Build history of the part. All positions in model axes, mm. Face numbers are marked on the shaded views. A direction names the side the tool comes from. Round coordinates to 2 decimals unless told otherwise and drop trailing zeros. Write each loop counter-clockwise with the first axis right and the second up, starting at its lowest first coordinate (ties: lowest second). Pieces come first, ordered by that corner, then holes. Notation, with made-up numbers: (40, -31) -> (99, -31) arc R30 cw to (99, -2) -> close; hole circle Ø5 at (21, -9.5). An arc over 180 degrees is marked (long way). Answer as CSV lines item,"result".
from build123d import *

# Parameters (mm, degrees)
BOSS_EXTRU_1_DEPTH = 10
ESQUISSE3_R        = 4.517940726
ESQUISSE3_R_2      = 2.1
BOSS_EXTRU_2_DEPTH = 4


with BuildPart() as part:
    # Esquisse1 → Boss.-Extru.1 (new body)
    with BuildSketch(Plane.XY):
        Polygon((-5.259154953, 5.14920934), (-7.281375044, 1.074544143), (-6.522357353, -3.410560394), (-3.27202084, -6.592946782), (1.228116422, -7.257051584), (5.259154953, -5.14920934), (7.281375044, -1.074544143), (6.522357353, 3.410560394), (3.27202084, 6.592946782), (-1.228116422, 7.257051584), align=None)
        Polygon((1.509357523, -3.811190523), (4.055266573, -0.598453303), (2.54590905, 3.21273722), (-1.509357523, 3.811190523), (-4.055266573, 0.598453303), (-2.54590905, -3.21273722), align=None, mode=Mode.SUBTRACT)
    extrude(amount=BOSS_EXTRU_1_DEPTH)

    # Esquisse3 → Boss.-Extru.2 (add)
    with BuildSketch(Plane.XY.offset(10)):
        Circle(ESQUISSE3_R)
        Circle(ESQUISSE3_R_2, mode=Mode.SUBTRACT)
    extrude(amount=-BOSS_EXTRU_2_DEPTH)


solid = part.part
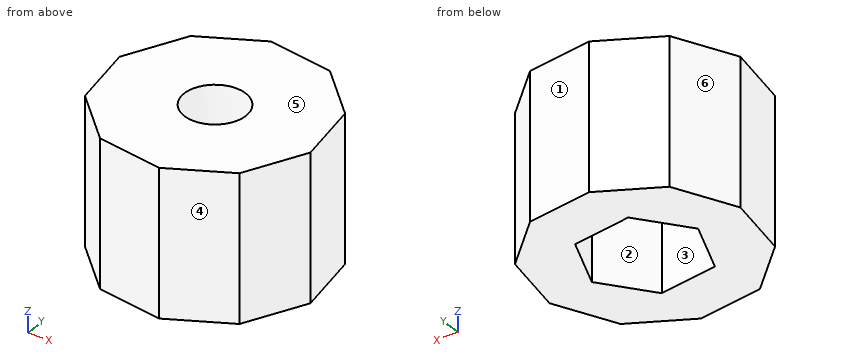
1. Drop flat-ended pins along their axis: pin 1 Ø1.5 at (x, z) = (-2.5, 6) entering from +Y; pin 2 Ø3 at (y, z) = (4.5, 1) entering from +X; pin 3 Ø6 at (x, z) = (4.5, 4) entering from +Y. Give the stop position or say it passes through.
Results found:
pin 1,"stops at y = 6.98"
pin 2,"stops at x = 6.59"
pin 3,"stops at y = 6.85"
2. Cut at A-A, the plane z = 8. Write the cut outline in (x, y), then the cut area to 3 significant figures.
Results found:
outline,"(-7.28, 1.07) -> (-6.52, -3.41) -> (-3.27, -6.59) -> (1.23, -7.26) -> (5.26, -5.15) -> (7.28, -1.07) -> (6.52, 3.41) -> (3.27, 6.59) -> (-1.23, 7.26) -> (-5.26, 5.15) -> close; hole circle Ø4.2 at (0, 0)"
area,"145 mm2"
3. Mould opens along Y. For the marked faces 3, 4, 5 and 6 say: +Y half, -Y half, draft (parallel to the pull), parting line (faces both ways), or undercut.
Results found:
face 3,"undercut"
face 4,"-Y half"
face 5,"draft"
face 6,"+Y half"
4. Cut at D-D, the plane z = 3.25. Write the cut outline in (x, y), then the cut area to 3 significant figures.
Results found:
outline,"(-7.28, 1.07) -> (-6.52, -3.41) -> (-3.27, -6.59) -> (1.23, -7.26) -> (5.26, -5.15) -> (7.28, -1.07) -> (6.52, 3.41) -> (3.27, 6.59) -> (-1.23, 7.26) -> (-5.26, 5.15) -> close; hole (-4.06, 0.6) -> (-2.55, -3.21) -> (1.51, -3.81) -> (4.06, -0.6) -> (2.55, 3.21) -> (-1.51, 3.81) -> close"
area,"116 mm2"
5. Which spindle directions (+Z, -Z, +X, -X, +Y, -Y) get a long thin tool onto all of the face, cutting with end or side? Do the marked faces 1 and 2. Say none if no direction does.
Results found:
face 1,"+Z, -Z, +X, +Y"
face 2,"-Z"
6. Cut at B-B, the plane x = 0. Write the cut outline in (y, z), then the cut area to 3 significant figures.
Results found:
outline,"(-7.08, 0) -> (-3.59, 0) -> (-3.59, 6) -> (-2.1, 6) -> (-2.1, 10) -> (-7.08, 10) -> close; (2.1, 6) -> (3.59, 6) -> (3.59, 0) -> (7.08, 0) -> (7.08, 10) -> (2.1, 10) -> close"
area,"81.7 mm2"
7. Cut at C-C, the plane y = 1.5. Write the cut outline in (x, z), then the cut area to 3 significant figures.
Results found:
outline,"(-7.07, 0) -> (-3.34, 0) -> (-3.34, 6) -> (-1.47, 6) -> (-1.47, 10) -> (-7.07, 10) -> close; (1.47, 6) -> (3.22, 6) -> (3.22, 0) -> (6.85, 0) -> (6.85, 10) -> (1.47, 10) -> close"
area,"88.0 mm2"
8. Probe line 1 along Y through (x, z) = (0, 7.65); line 2 along Z through (x, y) = (-2.25, -2.5); line 3 along X through (y, z) = (1.75, 7). List the from-to ranges inside material, lowest first.
Results found:
line 1,"y = -7.08 to -2.1, 2.1 to 7.08"
line 2,"z = 6 to 10"
line 3,"x = -6.95 to -1.16, 1.16 to 6.8"
